Geometry: final body of the model. Coordinates: model frame, mm. Face numbers are marked on the shaded views. Give positions to 0.01 mm unless a question says otherwise; leave off trailing zeros. Loops run counter-clockwise (first coordinate to the right, second up) from the corner with the lowest first, then second, coordinate; pieces in that order, holes last.
```python
from build123d import *

# Parameters (mm, degrees)
F0_R     = 77
F0_R_2   = 20
F1_DEPTH = 20
F3_D     = 10.5


with BuildPart() as f1:
    # F0 (on Front) → F1 (new body)
    with BuildSketch(Plane.XZ):
        Circle(F0_R)
        Circle(F0_R_2, mode=Mode.SUBTRACT)
    extrude(amount=F1_DEPTH)

    # F3 (through all)
    with Locations(Plane.XZ.offset(20)):
        with Locations((56.291651, -32.5), (65, 0), (56.291651, 32.5), (32.5, 56.291651), (0, 65), (-32.5, 56.291651), (-56.291651, 32.5), (-65, 0), (-56.291651, -32.5), (-32.5, -56.291651), (0, -65), (32.5, -56.291651)):
            Hole(F3_D / 2)


solid = f1.part
```
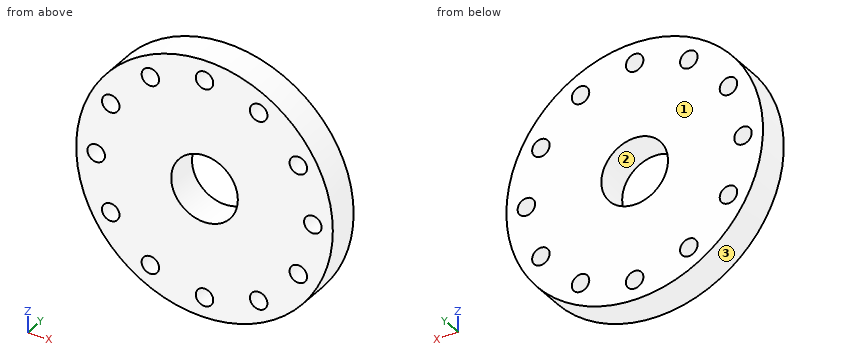
Q1. Pin query (flat end, axial travel): pin 1 Ø10 at (y, z) = (-14.5, 32.5) entering from +X; pin 2 Ø8 at (x, y) = (61.5, -4) entering from -Z; pin 3 Ø6.5 at (x, z) = (32.5, 56.29) entering from -Y; pin 4 Ø6 at (x, y) = (60.5, -2) entering from +Z. Return the tip coordinate at first contact, or that it passes through.
Q2. Section query D-D, the plane x = 65. Return loops of the section in (y, z), and give its area (3 significant figures).
Q3. Material intervals for probe 1 along Z at (x, y) = (0, -15.25); probe 2 along Z at (x, y) = (-57, -2.5); probe 3 along Z at (x, y) = (-29.5, -18.25), sorted ascending.
Q4. Section query B-B, the plane z = 0. Return loops of the section in (x, y).
Q5. Section query A-A, the plane x = 0. Return loops of the section in (y, z).
Q6. Section query C-C, the plane z = 65. Return loops of the section in (x, y).
Q7. Mould query, pull axis X, two halves, no side actions, for the marked faces 1, 2 and 3. Classes: +X half, -X half, draft (parallel to the pull), parting line (faces both ways), or undercut.
Resolved:
1. pin 1: stops at x = 71.92
1. pin 2: stops at z = -51.21
1. pin 3: passes through
1. pin 4: stops at z = 51.21
2. outline: (-20, -41.28) - (0, -41.28) - (0, -5.25) - (-20, -5.25) - close; (-20, 5.25) - (0, 5.25) - (0, 41.28) - (-20, 41.28) - close
2. area: 1,440 mm2
3. probe 1: z = -77 to -70.25, -59.75 to -20, 20 to 59.75, 70.25 to 77
3. probe 2: z = -51.77 to -37.7, -27.3 to 27.3, 37.7 to 51.77
3. probe 3: z = -71.12 to -60.6, -51.98 to 51.98, 60.6 to 71.12
4. outline: (-77, -20) - (-70.25, -20) - (-70.25, 0) - (-77, 0) - close; (-59.75, -20) - (-20, -20) - (-20, 0) - (-59.75, 0) - close; (20, -20) - (59.75, -20) - (59.75, 0) - (20, 0) - close; (70.25, -20) - (77, -20) - (77, 0) - (70.25, 0) - close
5. outline: (-20, -77) - (0, -77) - (0, -70.25) - (-20, -70.25) - close; (-20, -59.75) - (0, -59.75) - (0, -20) - (-20, -20) - close; (-20, 20) - (0, 20) - (0, 59.75) - (-20, 59.75) - close; (-20, 70.25) - (0, 70.25) - (0, 77) - (-20, 77) - close
6. outline: (-41.28, -20) - (-5.25, -20) - (-5.25, 0) - (-41.28, 0) - close; (5.25, -20) - (41.28, -20) - (41.28, 0) - (5.25, 0) - close
7. face 1: draft
7. face 2: undercut
7. face 3: parting line
